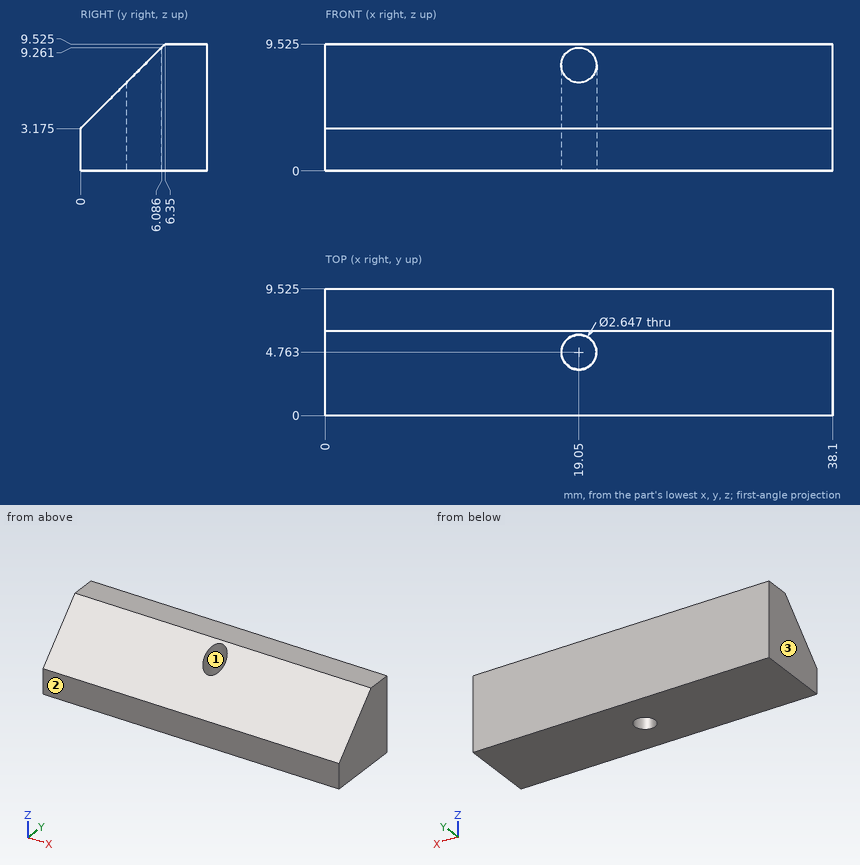
Source: three-view drawing plus pictorial views. Frame: mm from the lowest corner of the part. Round coordinates to 2 decimals unless told otherwise and drop trailing zeros. One line per item, written item: value.
(1) Line query: probe 1 along Y at (x, z) = (19.05, 2) (1 decimal); probe 2 along X at (y, z) = (4, 6); probe 3 along X at (y, z) = (4.5, 1.75). Output: solid intervals per line, ascending. Write a range as [from, to].
Result sheet:
probe 1: [0, 3.4], [6.1, 9.5]
probe 2: [0, 17.97], [20.13, 38.1]
probe 3: [0, 17.75], [20.35, 38.1]
(2) Pull-direction query (Y, two-part tool) for the marked faces 1, 2 and 3; classes: pulls with the +Y half, pulls with the -Y half, needs draft (parallel to the pull), parting line crosses it, or undercut.
Result sheet:
face 1: undercut
face 2: pulls with the -Y half
face 3: needs draft
(3) Pin query (flat end, axial travel): P1, Ø1, axis at x = 21, y = 2, coming from the -Z side; P2, Ø1.5, axis at x = 25.5, y = 2.5, coming from the +Z side (1 decimal). Return the tip coordinate at first contact, or that it passes through.
Result sheet:
P1: z = 0
P2: z = 6.4
